Work out the finished part from the listing and answer in its coordinate system (mm). Face numbers are marked on the shaded views. Give positions to 0.01 mm unless a question says otherwise; leave off trailing zeros. Order: outer loops, then holes, each group sorted by start corner. A loop starts at its lowest first (then second) coordinate and runs counter-clockwise, first axis right, second up. Notation, with made-up numbers: M -7.75,60 L 45.25,60 A26 ccw 45.25,85 Z; hole C 43,50.5 d11. An arc over 180 degrees is marked long. One line per item, written item: value.
from build123d import *

# Parameters (mm, degrees)
F0_R     = 19.05
F0_R_2   = 6.35
F1_DEPTH = 6.35
F2_R     = 5.08
F3_R     = 5.08


with BuildPart() as f1:
    # F0 (on Right) → F1 (new body, symmetric)
    with BuildSketch(Plane.YZ):
        Circle(F0_R)
        Circle(F0_R_2, mode=Mode.SUBTRACT)
    extrude(amount=F1_DEPTH, both=True)

    # F2
    f2_edges = [f1.edges().sort_by_distance(p)[0] for p in [
        (6.35, -19.05, 0),
    ]]
    fillet(f2_edges, radius=F2_R)

    # F3
    f3_edges = [f1.edges().sort_by_distance(p)[0] for p in [
        (-2.54, 19.05, 0),
        (1.27, -19.05, 0),
        (-6.35, -19.05, 0),
    ]]
    fillet(f3_edges, radius=F3_R)


solid = f1.part
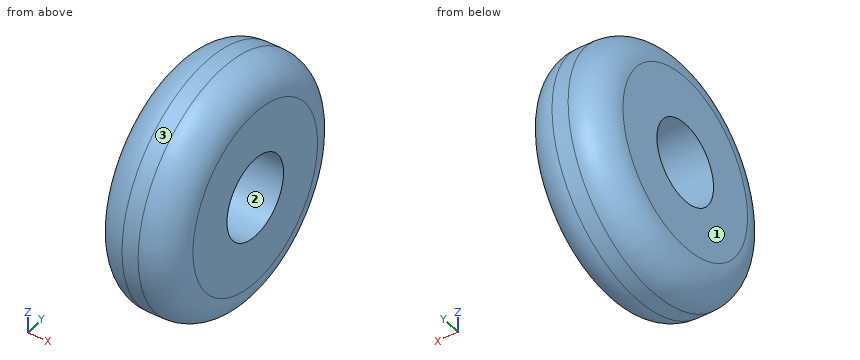
(1) Find the intervals of material crossed by probe 1 along Z at (x, y) = (-0.5, 0); probe 2 along Y at (x, z) = (0.25, 3); probe 3 along Z at (x, y) = (-3.25, 0), in increasing order. Write a range as from..to.
Findings:
probe 1: z = -19.05..-6.35, 6.35..19.05
probe 2: y = -18.81..-5.6, 5.6..18.81
probe 3: z = -18.65..-6.35, 6.35..18.65
(2) Given P1, Ø4, axis at x = 1, z = -3.5, coming from the -Y side; P2, Ø3, axis at x = -2.5, z = 10.5, coming from the -Y side; P3, Ø2, axis at x = -5, y = -9, coming from the -Z side; P4, Ø10, axis at y = 0, z = 0, coming from the +X side, each flat-ended and moving along its own axis, determine where each tip first touches the part or whether it passes through.
Findings:
P1: stops at y = -18.99
P2: stops at y = -16.68
P3: stops at z = -16.06
P4: passes through
(3) Section A-A, the plane y = 0 is taken. Give the vertices of the cut face in (x, z), then the cut area to 3 significant figures.
Findings:
outline: M -6.35,-13.97 A5.08 ccw -1.27,-19.05 L 1.27,-19.05 A5.08 ccw 6.35,-13.97 L 6.35,-6.35 L -6.35,-6.35 Z; M -6.35,6.35 L 6.35,6.35 L 6.35,13.97 A5.08 ccw 1.27,19.05 L -1.27,19.05 A5.08 ccw -6.35,13.97 Z
area: 300 mm^2
(4) Section C-C, the plane x = 0 is taken. Give the vertices of the cut face in (y, z).
Findings:
outline: C 0,0 d38.1; hole C 0,0 d12.7
(5) Determine the mould class of the marked faces 1, 2 and 3 for opening direction Z: pulls with the +Z half, pulls with the -Z half, needs draft (parallel to the pull), parting line crosses it, or undercut.
Findings:
face 1: needs draft
face 2: undercut
face 3: parting line crosses it
(6) Section D-D, the plane x = -5.5 is taken. Give the vertices of the cut face in (y, z), then the cut area to 3 significant figures.
Findings:
outline: C 0,0 d33.57; hole C 0,0 d12.7
area: 758 mm^2
